The listing builds one solid part. Answer for the finished solid, in the listing's coordinates (mm). A direction names the side the tool comes from. Round coordinates to 2 decimals unless told otherwise and drop trailing zeros.
Item 1: Find the intervals of material crossed by probe 1 along Y at (x, z) = (-415, 9); probe 2 along Y at (x, z) = (-350, 11.75); probe 3 along Y at (x, z) = (-300, 12), in increasing order.
Item 2: A tool of negligible diameter and unlimited length cuts with its end or side. For faces 1 (the face through (359, 0, 9)), 2 (the face through (-421, -2, 9)), from which of +Z, -Z, +X, -X, +Y, -Y can it reach the whole face along a straight path? Write none if from no direction.
Item 3: Each of these flat-tipped pins is pushed along its axis until it touches: pin 1 (7 mm diameter, centred on y = 50, z = 9, fed in from +X); pin 2 (4.5 mm diameter, centred on y = -75, z = 9, fed in from -X); pin 3 (4.5 mm diameter, centred on x = 0, y = -110, fed in from +Z); pin 4 (1 mm diameter, centred on y = 16.5, z = 2.5, fed in from +X). Where does it stop, or does it pass through?
```python
from build123d import *

# Parameters (mm, degrees)
SKETCH1_W                           = 842
SKETCH1_H                           = 250
BOSS_EXTRUDE1_DEPTH                 = 18
OTWORY_USTALAJ_CE_5_0MM1_D          = 5
OTWORY_USTALAJ_CE_6_0MM1_D          = 6
OTWORY_USTALAJ_CE_8_0MM1_D          = 8
OTWORY_USTALAJ_CE_5_0MM2_AT_2_COUNT = 2
OTWORY_USTALAJ_CE_5_0MM2_AT_2_PITCH = 150
WYTNIJ_WYCI_GNI_CIE1_DEPTH          = 440.533843976
OTW_R_8_0_8_1_AT_2_COUNT            = 2
OTW_R_8_0_8_1_AT_2_PITCH            = 100


with BuildPart() as part:
    # Sketch1 → Boss-Extrude1 (new body)
    with BuildSketch(Plane.XY):
        Rectangle(SKETCH1_W, SKETCH1_H)
    extrude(amount=BOSS_EXTRUDE1_DEPTH)

    # Otwory ustalające Ø5.0mm1 (through all)
    with Locations(Plane.XY.offset(18)):
        with Locations((-300, 110), (-300, 80), (-150, 110), (-150, 80), (0, 110), (0, 80), (150, 110), (150, 80), (300, 110), (300, 80), (-300, -80), (-300, -110), (-150, -80), (-150, -110), (0, -80), (0, -110), (150, -80), (150, -110), (300, -80), (300, -110)):
            Hole(OTWORY_USTALAJ_CE_5_0MM1_D / 2)

    # Otwory ustalające Ø6.0mm1 (through all)
    with Locations(Plane.XY.offset(18)):
        with Locations((-368, 23), (-368, -23), (333, 23), (346, 23), (333, -23), (346, -23)):
            Hole(OTWORY_USTALAJ_CE_6_0MM1_D / 2)

    # Otwory ustalające Ø8.0mm1 (through all)
    with Locations(Plane.XY.offset(18)):
        with Locations((-350, 60), (-175, 60), (0, 60), (175, 60), (350, 60), (350, -60), (175, -60), (0, -60), (-175, -60), (-350, -60)):
            Hole(OTWORY_USTALAJ_CE_8_0MM1_D / 2)

    # Szkic9 → Otwory ustalające Ø5.0mm2 (revolve, cut)
    with BuildSketch(Plane(origin=(421, 75, 9), x_dir=(0, 0, -1), z_dir=(0, 1, 0))):
        Polygon((0, 0), (0, 46.502151548), (2.5, 45), (2.5, 0), align=None)
    otwory_ustalaj_ce_5_0mm2 = revolve(axis=Axis((427.35, 75, 9), (-1, 0, 0)), mode=Mode.SUBTRACT)

    # Otwory ustalające Ø5.0mm2 at 2: Otwory ustalające Ø5.0mm2 ×2
    with Locations(*[(0, -i * OTWORY_USTALAJ_CE_5_0MM2_AT_2_PITCH, 0) for i in range(1, OTWORY_USTALAJ_CE_5_0MM2_AT_2_COUNT)]):
        add(otwory_ustalaj_ce_5_0mm2, mode=Mode.SUBTRACT)

    # Lustro1: Otwory ustalające Ø5.0mm2 across plane
    add(otwory_ustalaj_ce_5_0mm2.mirror(Plane.ZY), mode=Mode.SUBTRACT)

    # Lustro1 copy 1 sketch → Lustro1 copy 1 (revolve, cut)
    with BuildSketch(Plane(origin=(-421, -75, 9), x_dir=(0, 0, -1), z_dir=(0, 1, 0))):
        Polygon((0, 0), (0, -46.502151548), (2.5, -45), (2.5, 0), align=None)
    revolve(axis=Axis((-427.35, -75, 9), (-1, 0, 0)), mode=Mode.SUBTRACT)

    # Szkic10 → Wytnij-wyciągnięcie1 (cut, through all)
    with BuildSketch(Plane.XY.offset(18)):
        with BuildLine():
            Line((421, 30), (371, 30))
            ThreePointArc((371, 30), (362.514718626, 26.485281374), (359, 18))
            Line((359, 18), (359, -18))
            ThreePointArc((359, -18), (362.514718626, -26.485281374), (371, -30))
            Line((371, -30), (421, -30))
            Line((421, -30), (421, 30))
        make_face()
    extrude(amount=-WYTNIJ_WYCI_GNI_CIE1_DEPTH, mode=Mode.SUBTRACT)

    # Szkic11 → Otwór Ø8.0 (8)1 (revolve, cut)
    with BuildSketch(Plane(origin=(-421, 50, 9), x_dir=(0, 0, 1), z_dir=(0, 1, 0))):
        Polygon((0, 0), (0, 24.403442476), (4, 22), (4, 0), align=None)
    otw_r_8_0_8_1 = revolve(axis=Axis((-427.35, 50, 9), (1, 0, 0)), mode=Mode.SUBTRACT)

    # Otwór Ø8.0 (8)1 at 2: Otwór Ø8.0 (8)1 ×2
    with Locations(*[(0, -i * OTW_R_8_0_8_1_AT_2_PITCH, 0) for i in range(1, OTW_R_8_0_8_1_AT_2_COUNT)]):
        add(otw_r_8_0_8_1, mode=Mode.SUBTRACT)

    # Lustro2: Otwór Ø8.0 (8)1 across plane
    add(otw_r_8_0_8_1.mirror(Plane.ZY), mode=Mode.SUBTRACT)

    # Lustro2 copy 1 sketch → Lustro2 copy 1 (revolve, cut)
    with BuildSketch(Plane(origin=(421, -50, 9), x_dir=(0, 0, 1), z_dir=(0, 1, 0))):
        Polygon((0, 0), (0, -24.403442476), (4, -22), (4, 0), align=None)
    revolve(axis=Axis((427.35, -50, 9), (1, 0, 0)), mode=Mode.SUBTRACT)


solid = part.part
```
Check values:
1. probe 1: y = -125 to -77.5, -72.5 to -54, -46 to 46, 54 to 72.5, 77.5 to 125
1. probe 2: y = -125 to -64, -56 to 56, 64 to 125
1. probe 3: y = -125 to -112.5, -107.5 to -82.5, -77.5 to 77.5, 82.5 to 107.5, 112.5 to 125
2. face 1: +Z, -Z, +X
2. face 2: +Z, -Z, -X, +Y, -Y
3. pin 1: stops at x = 398.7
3. pin 2: stops at x = -375.85
3. pin 3: passes through
3. pin 4: stops at x = 359
